from build123d import *

# Parameters (mm, degrees)
SKETCH1_W            = 25
SKETCH1_H            = 25
BOSS_EXTRUDE1_DEPTH  = 3
SKETCH2_W            = 25
SKETCH2_H            = 3
BOSS_EXTRUDE2_DEPTH  = 22
BOSS_EXTRUDE3_DEPTH  = 2
BOSS_EXTRUDE4_DEPTH  = 2
M6_CLEARANCE_HOLE1_D = 6.6
M6_CLEARANCE_HOLE2_D = 6.6
FILLET1_R            = 1


with BuildPart() as part:
    # Sketch1 → Boss-Extrude1 (new body)
    with BuildSketch(Plane.XY):
        Rectangle(SKETCH1_W, SKETCH1_H)
    extrude(amount=BOSS_EXTRUDE1_DEPTH)

    # Sketch2 → Boss-Extrude2 (add)
    with BuildSketch(Plane.XY.offset(3)):
        with Locations((0, 11)):
            Rectangle(SKETCH2_W, SKETCH2_H)
    extrude(amount=BOSS_EXTRUDE2_DEPTH)

    # Sketch3 → Boss-Extrude3 (add)
    with BuildSketch(Plane(origin=(12.5, 0, 0), x_dir=(0, 0, -1), z_dir=(1, 0, 0))):
        Polygon((-25, 9.5), (-3, -12.5), (-3, 9.5), align=None)
    extrude(amount=-BOSS_EXTRUDE3_DEPTH)

    # Sketch4 → Boss-Extrude4 (add)
    with BuildSketch(Plane.ZY.offset(12.5)):
        Polygon((3, -12.5), (3, 9.5), (25, 9.5), align=None)
    extrude(amount=-BOSS_EXTRUDE4_DEPTH)

    # M6 Clearance Hole1 (through all)
    with Locations(Plane(origin=(0, 9.5, 0), x_dir=(-1, 0, 0), z_dir=(0, -1, 0))):
        with Locations((0, -12.5)):
            Hole(M6_CLEARANCE_HOLE1_D / 2)

    # M6 Clearance Hole2 (through all)
    with Locations(Plane.XY.offset(3)):
        with Locations((0, 0)):
            Hole(M6_CLEARANCE_HOLE2_D / 2)

    # Fillet1
    fillet1_edges = [part.edges().sort_by_distance(p)[0] for p in [
        (10.5, 9.5, 14),
        (10.5, -1.5, 3),
        (0, 9.5, 3),
        (-10.5, -1.5, 3),
        (-10.5, 9.5, 14),
    ]]
    fillet(fillet1_edges, radius=FILLET1_R)


solid = part.part
Read the model definition and answer for the solid it produces. Units are mm, in the model's axes. A direction names the side the tool comes from. Give positions to 0.01 mm unless a question says otherwise; leave off trailing zeros. Write each loop counter-clockwise with the first axis right and the second up, starting at its lowest first coordinate (ties: lowest second). Pieces come first, ordered by that corner, then holes. Notation, with made-up numbers: (12.25, 45) - (42.25, 45) arc R23 cw to (42.25, 77) - close; hole circle Ø2 at (-28, 10.25). An arc over 180 degrees is marked (long way). Return JSON: item names as keys, results as strings.
Q1. For faces 1 (the face through (-10.215, -1.853, 3.301)), 2 (the face through (-0.72, 11.02, 15.72)), determine the directions among +Z, -Z, +X, -X, +Y, -Y from which every point of the face is accessible in a straight line to the end or side of a thin tool.
Reply:
{"face 1": "+Z, -Y", "face 2": "+Y, -Y"}
Q2. A cutting plane is placed at B-B, the plane z = 12.5. Determine the outline of the cut face in (x, y).
Reply:
{"outline": "(-12.5, -3) - (-10.5, -3) - (-10.5, 8.5) arc R1 cw to (-9.5, 9.5) - (-3.3, 9.5) - (-3.3, 12.5) - (-12.5, 12.5) - close; (3.3, 9.5) - (9.5, 9.5) arc R1 cw to (10.5, 8.5) - (10.5, -3) - (12.5, -3) - (12.5, 12.5) - (3.3, 12.5) - close"}
Q3. A cutting plane is placed at D-D, the plane x = -6.75. Determine the outline of the cut face in (y, z).
Reply:
{"outline": "(-12.5, 0) - (12.5, 0) - (12.5, 25) - (9.5, 25) - (9.5, 4) arc R1 cw to (8.5, 3) - (-12.5, 3) - close"}
Q4. A cutting plane is placed at C-C, the plane x = 0. Determine the outline of the cut face in (y, z), and give its area (3 significant figures).
Reply:
{"outline": "(-12.5, 0) - (-3.3, 0) - (-3.3, 3) - (-12.5, 3) - close; (3.3, 0) - (12.5, 0) - (12.5, 9.2) - (9.5, 9.2) - (9.5, 4) arc R1 cw to (8.5, 3) - (3.3, 3) - close; (9.5, 15.8) - (12.5, 15.8) - (12.5, 25) - (9.5, 25) - close", "area": "102 mm²"}
Q5. Given P1, Ø5.5, axis at x = 0, y = 0, coming from the +Z side; P2, Ø5.5, axis at x = -3.5, y = -7, coming from the +Z side, each flat-ended and moving along its own axis, determine where each tip first touches the part or whether it passes through.
Reply:
{"P1": "through", "P2": "z = 3"}
Q6. For a pull along Y with two mould halves and no side action, classify faces 3 (the face through (2.43, 2.23, 1.48)), 4 (the face through (10.5, 3, 10)), 5 (the face through (0.133, 9.215, 3.301)) as released by +Y, released by -Y, zero draft, split by the parting line, or undercut.
Reply:
{"face 3": "undercut", "face 4": "zero draft", "face 5": "released by -Y"}
Q7. Consider line 1 along X through (y, z) = (8, 22.5); line 2 along X through (y, z) = (10.2, 12.5); line 3 along Z through (x, y) = (0, 10.5). Determine where each line is inside the solid, lowest interval first. Write a range as [from, to].
Reply:
{"line 1": "[-12.5, -10.5], [10.5, 12.5]", "line 2": "[-12.5, -3.3], [3.3, 12.5]", "line 3": "[0, 9.2], [15.8, 25]"}
Q8. A cutting plane is placed at A-A, the plane y = 0. Determine the outline of the cut face in (x, z), and give its area (3 significant figures).
Reply:
{"outline": "(-12.5, 0) - (-3.3, 0) - (-3.3, 3) - (-9.5, 3) arc R1 cw to (-10.5, 4) - (-10.5, 15.5) - (-12.5, 15.5) - close; (3.3, 0) - (12.5, 0) - (12.5, 15.5) - (10.5, 15.5) - (10.5, 4) arc R1 cw to (9.5, 3) - (3.3, 3) - close", "area": "106 mm²"}
